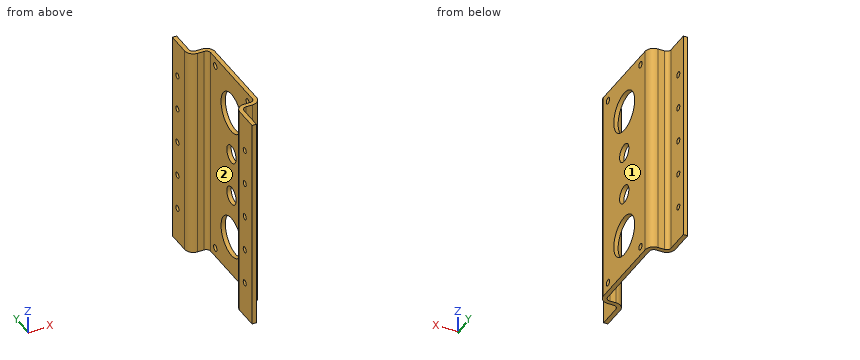
Autodesk Inventor part; units mm, degrees
ref_plane "YZ Plane" through (0, 0, 0) normal (1, 0, 0) x (0, 1, 0)
ref_plane "XZ Plane" through (0, 0, 0) normal (0, 1, 0) x (-1, 0, 0)
ref_plane "XY Plane" through (0, 0, 0) normal (0, 0, 1) x (1, 0, 0)
sketch "Sketch3" plane through (-13.672, 63.246, 0) normal (0, 1, 0) x (1, 0, 0)
  line L0 (10.624, 0) -> (10.624, 152.4)
  line L1 (0, 152.4) -> (10.624, 152.4)
  line L2 (0, 0) -> (0, 152.4)
  line L3 (10.624, 0) -> (0, 0)
  point P0 (13.672, 0)
  point P1 (5.312, 127)
  point P2 (5.312, 152.4)
  point P3 (5.312, 101.6)
  point P4 (5.312, 76.2)
  point P5 (5.312, 50.8)
  point P6 (5.312, 25.4)
  dimension "d28" = 25.4
  dimension "d31" = 25.4
sketch "Sketch1" plane through (0, 0, 0) normal (1, 0, 0) x (0, 1, 0)
  line L0 (0, 0) -> (57.15, 0)
  line L1 (57.15, 0) -> (57.15, -152.4)
  line L2 (57.15, -152.4) -> (0, -152.4)
  line L3 (0, -152.4) -> (0, 0)
  circle A0 centre (28.575, -28.575) radius 14.2875
  circle A1 centre (28.575, -60.325) radius 6.35
  circle A2 centre (28.575, -92.075) radius 6.35
  circle A3 centre (28.575, -123.825) radius 14.2875
  circle A4 centre (50.8, -6.35) radius 2.2479
  circle A5 centre (50.8, -146.05) radius 2.2479
  circle A6 centre (6.35, -146.05) radius 2.2479
  circle A7 centre (6.35, -6.35) radius 2.2479
  line L4 (50.8, -6.35) -> (6.35, -6.35) construction
  line L5 (6.35, -6.35) -> (6.35, -146.05) construction
  line L6 (6.35, -146.05) -> (50.8, -146.05) construction
  line L7 (50.8, -146.05) -> (50.8, -6.35) construction
  line L8 (57.15, 0) -> (69.85, 0)
  line L9 (69.85, 0) -> (69.85, -152.4)
  line L10 (69.85, -152.4) -> (57.15, -152.4)
  line L11 (57.15, -152.4) -> (57.15, 0)
  line L12 (0, -152.4) -> (-12.7, -152.4)
  line L13 (-12.7, -152.4) -> (-12.7, 0)
  line L14 (-12.7, 0) -> (0, 0)
  line L15 (0, 0) -> (0, -152.4)
  line L16 (28.575, -123.825) -> (28.575, -28.575)
  point P0 (28.575, -152.4)
  point P1 (28.575, -6.35)
  point P2 (28.575, 0)
  point P3 (50.8, -76.2)
  point P4 (57.15, -76.2)
  point P5 (57.15, -76.2)
  point P6 (28.575, -76.2)
  dimension "d0" = 57.15
  dimension "d1" = 152.4
  dimension "d2" = 31.75
  dimension "d3" = 31.75
  dimension "d4" = 31.75
  dimension "d6" = 28.575
  dimension "d7" = 12.7
  dimension "d8" = 28.575
  dimension "d11" = 4.4958
  dimension "d12" = 139.7
  dimension "d13" = 44.45
  dimension "d14" = 12.7
  dimension "d15" = 152.4
  dimension "d16" = 12.7
  dimension "d17" = 152.4
extrude "Plate2" add sketch "Sketch1" along normal blind 3.048 contours L0 L1 L2 L3
sketch "Sketch2" plane through (-3.048, 60.198, -152.4) normal (0, 1, 0) x (-1, 0, 0)
  line L0 (0, 152.4) -> (0, 0)
  line L1 (0, 0) -> (10.624, 0)
  line L2 (10.624, 0) -> (10.624, 152.4)
  line L3 (10.624, 152.4) -> (0, 152.4)
edge flange "Flange1" height 16.72 angle 90 thickness 3.048 bend radius 3.048 thickness toward (0, 1, 0) relief tear relief width 3.048 relief depth 1.524 corner gap 3.048 corner form 0 edges at (0, 57.15, -76.2) (0, 0, -76.2) wall of the first edge with corners at (-3.048, 60.198, 0) (-3.048, 60.198, -152.4) (-13.672, 60.198, -152.4) (-13.672, 60.198, 0)
bend "Bend1"
corner "Corner1"
sketch "Sketch4" plane through (-10.624, -3.048, -152.4) normal (-1, 0, 0) x (0, -1, 0)
  line L0 (0, 152.4) -> (0, 0)
  line L1 (0, 0) -> (23.048, 0)
  line L2 (23.048, 0) -> (23.048, 152.4)
  line L3 (23.048, 152.4) -> (0, 152.4)
edge flange "Flange2" height 20 angle 90 thickness 3.048 bend radius 3.048 thickness toward (-1, 0, 0) relief tear relief width 3.048 relief depth 1.524 corner gap 3.048 corner form 0 edges at (-13.672, -6.096, -76.2) (-13.672, 63.246, -76.2) wall of the first edge with corners at (-10.624, -3.048, 0) (-10.624, -3.048, -152.4) (-10.624, -26.096, -152.4) (-10.624, -26.096, 0)
bend "Bend2"
corner "Corner2"
sketch "Sketch5" plane through (-10.624, -26.096, 0) normal (1, 0, 0) x (0, 0, -1)
  line L0 (152.4, 16.952) -> (152.4, 0)
  line L1 (0, 0) -> (152.4, 0)
  point P0 (0, 26.096)
  point P1 (127, 10)
  point P2 (101.6, 10)
  point P3 (76.2, 10)
  point P4 (50.8, 10)
  point P5 (25.4, 10)
  point P6 (50.8, 102.39)
  point P7 (25.4, 102.39)
  point P8 (76.2, 102.39)
  point P9 (101.6, 102.39)
  point P10 (127, 102.39)
  dimension "d53" = 25.4
  dimension "d54" = 10
  dimension "d57" = 25.4
  dimension "d74" = 92.39
hole "Hole2" at (-10.624, -16.096, -127) at (-10.624, -16.096, -101.6) at (-10.624, -16.096, -76.2) at (-10.624, -16.096, -50.8) at (-10.624, -16.096, -25.4) at (-10.624, 76.294, -25.4) at (-10.624, 76.294, -50.8) at (-10.624, 76.294, -76.2) at (-10.624, 76.294, -101.6) at (-10.624, 76.294, -127) direction (-1, 0, 0) diameter 4.134 end through all
equation "\"d10\" = Thickness"
equation "\"d18\" = BendReliefWidth"
equation "\"d19\" = BendReliefDepth"
equation "\"d20\" = MinimumRemnant"
equation "\"d21\" = TransitionRadius"
equation "\"d24\" = BendRadius"
equation "\"d25\" = CornerReliefSize"
equation "\"d26\" = GapSize"
equation "\"d27\" = JacobiRadiusSize"
equation "\"d43\" = BendReliefWidth"
equation "\"d44\" = BendReliefDepth"
equation "\"d45\" = MinimumRemnant"
equation "\"d46\" = TransitionRadius"
equation "\"d49\" = BendRadius"
equation "\"d50\" = CornerReliefSize"
equation "\"d51\" = GapSize"
equation "\"d52\" = JacobiRadiusSize"
equation "\"BendRadius\" = Thickness"
equation "\"BendReliefWidth\" = Thickness"
equation "\"BendReliefDepth\" = 0.5 * Thickness"
equation "\"CornerReliefSize\" = 4 * Thickness"
equation "\"MinimumRemnant\" = 2 * Thickness"
equation "\"TransitionRadius\" = BendRadius"
equation "\"JacobiRadiusSize\" = BendRadius"
equation "\"GapSize\" = Thickness"
properties part number "CH-1-01-RearGearboxHousingMotorSide" material "Steel, Alloy"
Source: CAD feature listing. Evaluate the final solid. Frame: model axes, mm. Face numbers are marked on the shaded views. Coordinates: 2 decimals unless noted, no trailing zeros. Loops run counter-clockwise (first coordinate to the right, second up) from the corner with the lowest first, then second, coordinate; pieces in that order, holes last. Notation, with made-up numbers: M 9.5,7.25 L 49.5,7.25 A17 ccw 49.5,11.25 Z; hole C 61,30.5 d5. An arc over 180 degrees is marked long. Answer in a Markdown table with one row per item.
Q1. Section D-D on z = -127. State how many separate pieces and enclosed holes the cut face has, plus the area to 3 significant figures.
Answers below:
| item | result |
|---|---|
| separate pieces | 4 |
| enclosed holes | 0 |
| area | 283 mm^2 |
Q2. First-contact query: pin 1 (2 mm diameter, centred on x = -0.5, z = -52.5, fed in from +Y); pin 2 (5 mm diameter, centred on x = -7.5, z = -129.5, fed in from +Y); pin 3 (5 mm diameter, centred on x = -4.5, z = -91.5, fed in from -Y). Flat tips, straight axial feed; report the tip coordinate or a pass-through.
Answers below:
| item | result |
|---|---|
| pin 1 | stops at y = 63.05 |
| pin 2 | stops at y = 64.45 |
| pin 3 | stops at y = -6.1 |
Q3. Draft query along Y for the marked faces 1 and 2. Return one class per face: pulls with the +Y half, pulls with the -Y half, needs draft (parallel to the pull), parting line crosses it, or undercut.
Answers below:
| item | result |
|---|---|
| face 1 | needs draft |
| face 2 | undercut |
Q4. Section C-C on z = -37.5. Return the cut outline in (x, y), plus the area to 3 significant figures.
Answers below:
| item | result |
|---|---|
| outline | M -13.67,-26.1 L -10.62,-26.1 L -10.62,-9.14 A3.05 cw -7.58,-6.1 L -3.05,-6.1 A6.1 ccw 3.05,0 L 3.05,17.42 L 0,17.42 L 0,0 A3.05 cw -3.05,-3.05 L -7.58,-3.05 A6.1 ccw -13.67,-9.14 Z; M -13.67,66.29 A6.1 ccw -7.58,60.2 L -3.05,60.2 A3.05 cw 0,57.15 L 0,39.73 L 3.05,39.73 L 3.05,57.15 A6.1 ccw -3.05,63.25 L -7.58,63.25 A3.05 cw -10.62,66.29 L -10.62,83.25 L -13.67,83.25 Z |
| area | 325 mm^2 |
Q5. Section A-A on y = 50.8. Return the cut outline in (x, z).
Answers below:
| item | result |
|---|---|
| outline | M 0,-152.4 L 3.05,-152.4 L 3.05,-148.3 L 0,-148.3 Z; M 0,-143.8 L 3.05,-143.8 L 3.05,-8.6 L 0,-8.6 Z; M 0,-4.1 L 3.05,-4.1 L 3.05,0 L 0,0 Z |
Q6. Section B-B on z = -6.35. Return the cut outline in (x, y), plus the area to 3 significant figures.
Answers below:
| item | result |
|---|---|
| outline | M -13.67,-26.1 L -10.62,-26.1 L -10.62,-9.14 A3.05 cw -7.58,-6.1 L -3.05,-6.1 A6.1 ccw 3.05,0 L 3.05,4.1 L 0,4.1 L 0,0 A3.05 cw -3.05,-3.05 L -7.58,-3.05 A6.1 ccw -13.67,-9.14 Z; M -13.67,66.29 A6.1 ccw -7.58,60.2 L -3.05,60.2 A3.05 cw 0,57.15 L 0,53.05 L 3.05,53.05 L 3.05,57.15 A6.1 ccw -3.05,63.25 L -7.58,63.25 A3.05 cw -10.62,66.29 L -10.62,83.25 L -13.67,83.25 Z; M 0,8.6 L 3.05,8.6 L 3.05,48.55 L 0,48.55 Z |
| area | 365 mm^2 |
Q7. Ray query, probe 1 along Y at (x, z) = (-5.5, -132.5); probe 2 along Y at (x, z) = (-11.8, -101.6); probe 3 along Y at (x, z) = (-12.2, -25.4). Return the intervals inside material, ascending. Write a range as from..to.
Answers below:
| item | result |
|---|---|
| probe 1 | y = -6.1..-3.05, 60.2..63.25 |
| probe 2 | y = -26.1..-18.16, -14.03..-4.75, 61.9..74.23, 78.36..83.25 |
| probe 3 | y = -26.1..-18.16, -14.03..-5.17, 62.32..74.23, 78.36..83.25 |
